The model under review builds one solid part; all positions refer to its coordinate system, in mm. Face numbers are marked on the shaded views. A direction names the side the tool comes from. Give positions to 0.01 mm unless a question says otherwise; leave off trailing zeros. Order: outer loops, then holes, each group sorted by start corner. A loop starts at its lowest first (then second) coordinate and runs counter-clockwise, first axis right, second up. Notation, with made-up numbers: (-10, -36.75) - (6, -36.75) arc R24 ccw to (6, -6.75) - close; hole circle Ø2 at (54, 32). An arc over 180 degrees is marked (long way). Put each result on its own line as item: value.
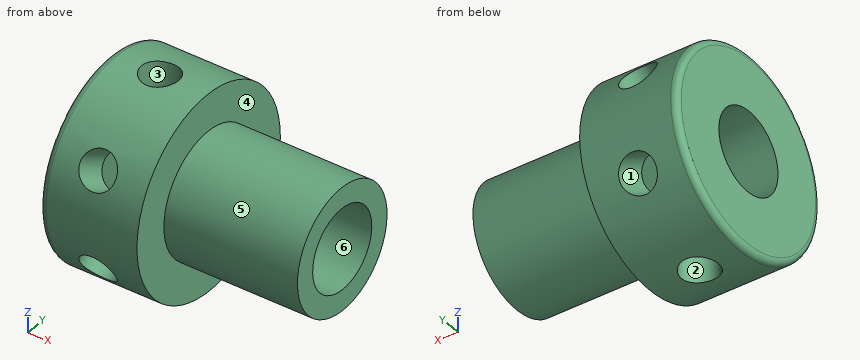
Autodesk Inventor part; units mm, degrees
ref_plane "Arbeitsebene1" through (0, 0, 8) normal (0, 0, 1) x (1, 0, 0)
ref_plane "YZ Plane" through (0, 0, 0) normal (1, 0, 0) x (0, 1, 0)
ref_plane "XZ Plane" through (0, 0, 0) normal (0, 1, 0) x (-1, 0, 0)
sketch "Skizze1" plane through (0, 0, 0) normal (1, 0, 0) x (0, 1, 0)
  circle A0 centre (0, 0) radius 8
  dimension "d0" = 16
extrude "Extrusion1" add sketch "Skizze1" along normal blind 8
sketch "Skizze2" plane through (8, 0, 0) normal (1, 0, 0) x (0, 0, -1)
  circle A0 centre (0, 0) radius 5
  dimension "d3" = 10
extrude "Extrusion2" add sketch "Skizze2" along normal blind 11
thread "Gewinde1"
ref_plane "Arbeitsebene1" through (0, 0, 8) normal (0, 0, 1) x (1, 0, 0)
sketch "Skizze3" plane through (0, 0, 8) normal (0, 0, 1) x (1, 0, 0)
  circle A0 centre (4, 0) radius 1.5
  point P0 (0, 0)
  dimension "d9" = 3
extrude "Extrusion3" cut sketch "Skizze3" against normal blind 3
sketch "Skizze4" plane through (19, 0, 0) normal (1, 0, 0) x (0, 0, -1)
  point P0 (0, 0)
hole "Bohrung1" at (19, 0, 0) direction (-1, 0, 0) diameter 6.6 depth 19
pattern_circular "Runde Anordnung1" count 6 over 360 about axis through (0, 0, 0) along (1, 0, 0) of "Extrusion3"
fillet "Rundung1" radius 0.5 1 edges at (0, -8, 0)
properties part number "sf_Piston_Rod_Gland_1"
(1) Take a section at D-D, the plane x = 7. Write out the cut boundary in (y, z).
The answers:
outline: circle Ø16 at (0, 0); hole circle Ø6.6 at (0, 0)
(2) Clearance check with flat-ended pins moving along their axes: pin 1 Ø2 at (x, z) = (9.5, 4.5) entering from -Y; pin 2 Ø3 at (x, y) = (3, -3) entering from +Z; pin 3 Ø0.9 at (x, y) = (4.5, -0.5) entering from -Z. State where each tip first meets the part, or that it passes through.
The answers:
pin 1: y = -3.57
pin 2: z = 7.86
pin 3: z = -5
(3) Take a section at A-A, the plane y = 0. Write out the cut boundary in (x, z).
The answers:
outline: (0, -7.5) arc R0.5 ccw to (0.5, -8) - (2.5, -8) - (2.5, -5) - (5.5, -5) - (5.5, -8) - (8, -8) - (8, -5) - (19, -5) - (19, -3.3) - (0, -3.3) - close; (0, 3.3) - (19, 3.3) - (19, 5) - (8, 5) - (8, 8) - (5.5, 8) - (5.5, 5) - (2.5, 5) - (2.5, 8) - (0.5, 8) arc R0.5 ccw to (0, 7.5) - close
(4) Take a section at B-B, the plane z = 0. Write out the cut boundary in (x, y), then the cut area to 3 significant figures.
The answers:
outline: (0, -7.5) arc R0.5 ccw to (0.5, -8) - (8, -8) - (8, -5) - (19, -5) - (19, -3.3) - (0, -3.3) - close; (0, 3.3) - (19, 3.3) - (19, 5) - (8, 5) - (8, 8) - (0.5, 8) arc R0.5 ccw to (0, 7.5) - close
area: 112 mm^2
(5) The part is to be moulded in two halves that separate along Y. For the marked faces 4, 5 and 6, say which applies: pulls with the +Y half, pulls with the -Y half, needs draft (parallel to the pull), parting line crosses it, or undercut.
The answers:
face 4: needs draft
face 5: parting line crosses it
face 6: undercut
(6) For the marked faces 1, 2 and 3, list the 3-axis set-ups (+Z, -Z, +X, -X, +Y, -Y) from which the entire face can be reached by the end or side of a thin tool; tool diameter is ignored.
The answers:
face 1: none
face 2: -Z
face 3: +Z
(7) Wall thickness on L1, parallel to Y at x = 10, z = 0; L2, parallel to X at y = 0, z = -6.6; L3, parallel to Z at x = 3.25, y = -4.5: over which ranges is each line inside the solid? List them lowest first.
The answers:
L1: -5 to -3.3, 3.3 to 5
L2: 0 to 2.5, 5.5 to 8
L3: -6.61 to -4.1, -2.21 to 2.21, 4.1 to 6.61
(8) Take a section at C-C, the plane x = 4. Write out the cut boundary in (y, z), then the cut area to 3 significant figures.
The answers:
outline: (-7.56, -2.63) - (-5.08, -1.2) - (-3.58, -3.8) - (-6.06, -5.23) arc R8 ccw to (-1.5, -7.86) - (-1.5, -5) - (1.5, -5) - (1.5, -7.86) arc R8 ccw to (6.06, -5.23) - (3.58, -3.8) - (5.08, -1.2) - (7.56, -2.63) arc R8 ccw to (7.56, 2.63) - (5.08, 1.2) - (3.58, 3.8) - (6.06, 5.23) arc R8 ccw to (1.5, 7.86) - (1.5, 5) - (-1.5, 5) - (-1.5, 7.86) arc R8 ccw to (-6.06, 5.23) - (-3.58, 3.8) - (-5.08, 1.2) - (-7.56, 2.63) arc R8 ccw to start; hole circle Ø6.6 at (0, 0)
area: 114 mm^2
